from build123d import *

# Parameters (mm, degrees)
F0_W      = 54
F0_H      = 50
F0_R      = 1
F1_DEPTH  = 1.5
F2_W      = 1.5
F2_H      = 50
F3_DEPTH  = 28
F4_W      = 50
F4_H      = 1.5
F5_DEPTH  = 13
F6_R      = 1
F7_DEPTH  = 1.5
F9_R      = 6.5
F10_DEPTH = 57.001
F11_R     = 17.5
F12_DEPTH = 1.5


with BuildPart() as f1:
    # F0 (on Top) → F1 (new body)
    with BuildSketch(Plane.XY):
        Rectangle(F0_W, F0_H)
        with Locations((-23.5, -21.5)):
            Circle(F0_R, mode=Mode.SUBTRACT)
        with Locations((23.5, -21.5)):
            Circle(F0_R, mode=Mode.SUBTRACT)
        with Locations((-23.5, 21.5)):
            Circle(F0_R, mode=Mode.SUBTRACT)
        with Locations((23.5, 21.5)):
            Circle(F0_R, mode=Mode.SUBTRACT)
    extrude(amount=F1_DEPTH)

    # F2 (on Top) → F3 (join)
    with BuildSketch(Plane.XY):
        with Locations((27.75, 0)):
            Rectangle(F2_W, F2_H)
    extrude(amount=F3_DEPTH)

    # F4 (on face) → F5 (join)
    with BuildSketch(Plane(origin=(27, 0, 0), x_dir=(0, -1, 0), z_dir=(-1, 0, 0))):
        with Locations((0, 27.25)):
            Rectangle(F4_W, F4_H)
    extrude(amount=F5_DEPTH)

    # F6 (on face) → F7 (cut, through all)
    with BuildSketch(Plane.XY.offset(28)):
        with Locations((20, 22)):
            Circle(F6_R)
        with Locations((20, 7)):
            Circle(F6_R)
    extrude(amount=-F7_DEPTH, mode=Mode.SUBTRACT)

    # F8: F1 across plane


with BuildPart() as f1_1:
    add(f1.part)
    add(f1.part.mirror(Plane.YZ))

    # F9 (on face) → F10 (cut, through all)
    with BuildSketch(Plane(origin=(-28.5, 0, 0), x_dir=(0, -1, 0), z_dir=(-1, 0, 0))):
        with Locations((-13, 14)):
            Circle(F9_R)
        with Locations((13, 14)):
            Circle(F9_R)
    extrude(amount=-F10_DEPTH, mode=Mode.SUBTRACT)

    # F11 (on face) → F12 (cut, through all)
    with BuildSketch(Plane(origin=(0, 0, 0), x_dir=(1, 0, 0), z_dir=(0, 0, -1))):
        Circle(F11_R)
    extrude(amount=-F12_DEPTH, mode=Mode.SUBTRACT)


solid = f1_1.part
Work out the finished part from the listing and answer in its coordinate system (mm). A direction names the side the tool comes from. Round coordinates to 2 decimals unless told otherwise and drop trailing zeros. Loops run counter-clockwise (first coordinate to the right, second up) from the corner with the lowest first, then second, coordinate; pieces in that order, holes last. Notation, with made-up numbers: (-11, 5.25) - (24, 5.25) arc R18 ccw to (24, 40.25) - close; hole circle Ø8 at (12.5, 12.5). An arc over 180 degrees is marked (long way). One line per item, written item: value.
Q1. Find section B-B on z = 14. Give the vertices of the cut face in (x, y).
Check values:
outline: (-28.5, -25) - (-27, -25) - (-27, -19.5) - (-28.5, -19.5) - close; (-28.5, -6.5) - (-27, -6.5) - (-27, 6.5) - (-28.5, 6.5) - close; (-28.5, 19.5) - (-27, 19.5) - (-27, 25) - (-28.5, 25) - close; (27, -25) - (28.5, -25) - (28.5, -19.5) - (27, -19.5) - close; (27, -6.5) - (28.5, -6.5) - (28.5, 6.5) - (27, 6.5) - close; (27, 19.5) - (28.5, 19.5) - (28.5, 25) - (27, 25) - close
Q2. Find section C-C on x = -15. Give the vertices of the cut face in (y, z), and give its area (3 significant figures).
Check values:
outline: (-25, 0) - (-9.01, 0) - (-9.01, 1.5) - (-25, 1.5) - close; (-25, 26.5) - (25, 26.5) - (25, 28) - (-25, 28) - close; (9.01, 0) - (25, 0) - (25, 1.5) - (9.01, 1.5) - close
area: 123 mm2
Q3. Find section D-D on x = 9.5. Give the vertices of the cut face in (y, z), and give its area (3 significant figures).
Check values:
outline: (-25, 0) - (-14.7, 0) - (-14.7, 1.5) - (-25, 1.5) - close; (14.7, 0) - (25, 0) - (25, 1.5) - (14.7, 1.5) - close
area: 30.9 mm2
Q4. This flat-tipped pin is pushed along its axis until it touches: pin 1 Ø1.6 at (x, y) = (-23.5, 21.5) entering from -Z. Where does it stop, or does it pass through?
Check values:
pin 1: z = 26.5
Q5. For faces 1 (the flat face through (14, 0, 27)), 2 (the flat face through (-21, 0, 26.5)), 3 (the cylindrical face through (-23.717, -22.476, 0.74)), 4 (the cylindrical face through (-20, 21, 27)), determine the directions among +Z, -Z, +X, -X, +Y, -Y from which every point of the face is accessible in a straight line to the end or side of a thin tool.
Check values:
face 1: +Z, +Y, -Y
face 2: +Y, -Y
face 3: -Z
face 4: +Z
Q6. Straight lines are drawn through the part: probe 1 along X at (y, z) = (-21.5, 0.4); probe 2 along Y at (x, z) = (23.5, 0.4); probe 3 along X at (y, z) = (-7, 19.75). For each, find the intervals that lie inside material, in ascending order.
Check values:
probe 1: -28.5 to -24.5, -22.5 to 22.5, 24.5 to 28.5
probe 2: -25 to -22.5, -20.5 to 20.5, 22.5 to 25
probe 3: -28.5 to -27, 27 to 28.5
Q7. Find section A-A on y = 0. Give the vertices of the cut face in (x, z), and give its area (4 significant figures).
Check values:
outline: (-28.5, 0) - (-17.5, 0) - (-17.5, 1.5) - (-27, 1.5) - (-27, 26.5) - (-14, 26.5) - (-14, 28) - (-28.5, 28) - close; (14, 26.5) - (27, 26.5) - (27, 1.5) - (17.5, 1.5) - (17.5, 0) - (28.5, 0) - (28.5, 28) - (14, 28) - close
area: 151.5 mm2
Q8. The mould has two halves that part along Y. Classify faces 5 (the cylindrical face through (-19.263, 7.676, 27.26)), 6 (the flat face through (0, 25, 1)), 7 (the cylindrical face through (-23.717, 20.524, 0.74)), 8 (the flat face through (-21, 0, 28)): +Y half, -Y half, draft (parallel to the pull), parting line (faces both ways), or undercut.
Check values:
face 5: undercut
face 6: +Y half
face 7: undercut
face 8: draft
